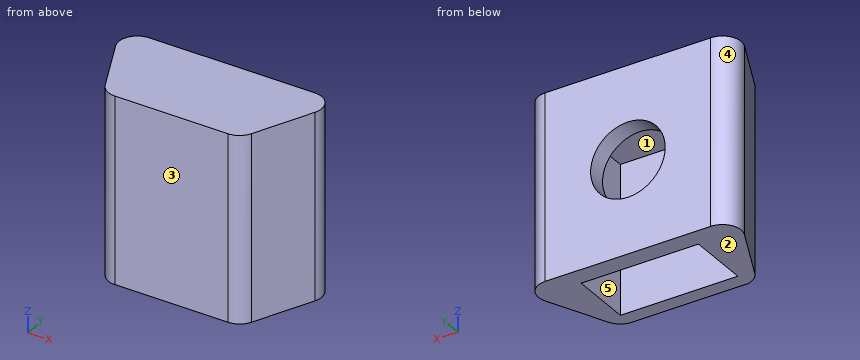
```python
from build123d import *

# Parameters (mm, degrees)
SKETCH1_W           = 6.3
SKETCH1_H           = 3.3
BOSS_EXTRUDE1_DEPTH = 8
BOSS_EXTRUDE2_DEPTH = 2
SKETCH2_R           = 2
CUT_EXTRUDE1_DEPTH  = 1
FILLET1_R           = 1


with BuildPart() as part:
    # Sketch1 → Boss-Extrude1 (new body)
    with BuildSketch(Plane.XY):
        Polygon((-6, 2.65), (6, 2.65), (3.663445075, -2.45), (-3.663445075, -2.45), align=None)
        Rectangle(SKETCH1_W, SKETCH1_H, mode=Mode.SUBTRACT)
    extrude(amount=-BOSS_EXTRUDE1_DEPTH)

    # Sketch1<2> → Boss-Extrude2 (add)
    with BuildSketch(Plane.XY):
        Polygon((-6, 2.65), (6, 2.65), (3.663445075, -2.45), (-3.663445075, -2.45), align=None)
    extrude(amount=BOSS_EXTRUDE2_DEPTH)

    # Sketch2 → Cut-Extrude1 (cut)
    with BuildSketch(Plane(origin=(0, 2.65, 0), x_dir=(1, 0, 0), z_dir=(0, 1, 0))):
        with Locations(Location((0, 3, 0), (0, 0, 180))):
            Circle(SKETCH2_R)
    extrude(amount=-CUT_EXTRUDE1_DEPTH, mode=Mode.SUBTRACT)

    # Fillet1
    fillet1_edges = [part.edges().sort_by_distance(p)[0] for p in [
        (-6, 2.65, -3),
        (6, 2.65, -3),
        (3.663445075, -2.45, -3),
        (-3.663445075, -2.45, -3),
    ]]
    fillet(fillet1_edges, radius=FILLET1_R)


solid = part.part
```
Read the model definition and answer for the solid it produces. Units are mm, in the model's axes. Face numbers are marked on the shaded views. A direction names the side the tool comes from. Coordinates: 2 decimals unless noted, no trailing zeros. Loops run counter-clockwise (first coordinate to the right, second up) from the corner with the lowest first, then second, coordinate; pieces in that order, holes last. Notation, with made-up numbers: (34.5, 47) - (50.5, 47) arc R29 cw to (50.5, 78) - close; hole circle Ø7 at (18, -9.5). An arc over 180 degrees is marked (long way). Answer in a Markdown table with one row per item.
1. Straight lines are drawn through the part: line 1 (Y direction, x = -2, z = -5); line 2 (Z direction, x = 0, y = 2.4); line 3 (Y direction, x = 0.75, z = -3.75). For each, find the intervals that lie inside material, in ascending order.
Conclusion:
| item | result |
|---|---|
| line 1 | y = -2.45 to -1.65, 1.65 to 2.65 |
| line 2 | z = -8 to -5, -1 to 2 |
| line 3 | y = -2.45 to -1.65 |
2. Find section B-B, the plane z = -6.5. Write down the section's boundary in (x, y).
Conclusion:
| item | result |
|---|---|
| outline | (-5.35, 1.23) - (-3.93, -1.87) arc R1 ccw to (-3.02, -2.45) - (3.02, -2.45) arc R1 ccw to (3.93, -1.87) - (5.35, 1.23) arc R1 ccw to (4.44, 2.65) - (-4.44, 2.65) arc R1 ccw to start; hole (-3.15, -1.65) - (3.15, -1.65) - (3.15, 1.65) - (-3.15, 1.65) - close |
3. Find section A-A, the plane x = 0. Write down the section's boundary in (y, z).
Conclusion:
| item | result |
|---|---|
| outline | (-2.45, -8) - (-1.65, -8) - (-1.65, 0) - (1.65, 0) - (1.65, -1) - (2.65, -1) - (2.65, 2) - (-2.45, 2) - close; (1.65, -8) - (2.65, -8) - (2.65, -5) - (1.65, -5) - close |
4. Given pin 1 (1 mm diameter, centred on y = 0, z = -3, fed in from -X) (3 decimals); pin 2 (1 mm diameter, centred on y = 0, z = -5.5, fed in from +X) (3 decimals); pin 3 (3 mm diameter, centred on y = -2, z = -6.5, fed in from +X), each flat-ended and moving along its own axis, determine where each tip first touches the part or whether it passes through.
Conclusion:
| item | result |
|---|---|
| pin 1 | stops at x = -5.015 |
| pin 2 | stops at x = 5.015 |
| pin 3 | stops at x = 4.56 |
5. Determine the mould class of the marked faces 3, 4 and 5 for opening direction Y: +Y half, -Y half, draft (parallel to the pull), parting line (faces both ways), or undercut.
Conclusion:
| item | result |
|---|---|
| face 3 | -Y half |
| face 4 | parting line |
| face 5 | undercut |
6. Which of the six approach directions +Z, -Z, +X, -X, +Y, -Y give full straight-line access (tool end or side, diameter ignored) to the marked faces 1 and 2?
Conclusion:
| item | result |
|---|---|
| face 1 | -Z |
| face 2 | -Z, +X, -X, +Y, -Y |
7. Find section D-D, the plane y = 0.7. Write down the section's boundary in (x, z).
Conclusion:
| item | result |
|---|---|
| outline | (-5.11, -8) - (-3.15, -8) - (-3.15, 0) - (3.15, 0) - (3.15, -8) - (5.11, -8) - (5.11, 2) - (-5.11, 2) - close |
8. Find section C-C, the plane x = -2.25. Write down the section's boundary in (y, z), then the cut area to 3 significant figures.
Conclusion:
| item | result |
|---|---|
| outline | (-2.45, -8) - (-1.65, -8) - (-1.65, 0) - (1.65, 0) - (1.65, -8) - (2.65, -8) - (2.65, 2) - (-2.45, 2) - close |
| area | 24.6 mm² |
